Check sheet for the drawn part. Datum: minimum x, y, z corner. Units: mm. Give positions to 0.01 mm unless a question says otherwise; leave off trailing zeros. Write each loop counter-clockwise with the first axis right and the second up, starting at its lowest first coordinate (ties: lowest second). Pieces come first, ordered by that corner, then holes. Notation, with made-up numbers: (-20.75, 24.5) -> (-9.75, 24.5) arc R18 ccw to (-9.75, 56.5) -> close; hole circle Ø3 at (68.5, 31.25). An arc over 180 degrees is marked (long way). Answer as CSV lines item,"result". Start each with the question number.
1) Sectioned sample at B-B on x = 38. Record the cut outline in (y, z), and give its area (3 significant figures).
2) Sectioned sample at A-A on z = 31. Record the cut outline in (x, y).
3) Material ranges on L1, parallel to X at y = 4.4, z = 39; L2, parallel to Z at x = 42.5, y = 3.35; L3, parallel to Z at x = 30.5, y = 1.75, recorded low to high.
4) Gauge pin test, flat ends, axial feed: pin 1 Ø1.5 at (x, y) = (46.5, 1.5) entering from +Z; pin 2 Ø1 at (y, z) = (2, 7.5) entering from -X; pin 3 Ø1.5 at (x, y) = (25, 2) entering from +Z. Record the tip position at first contact, or that the pin passes through.
5) Sectioned sample at C-C on y = 2.1. Record the cut outline in (x, z), and give its area (3 significant figures).
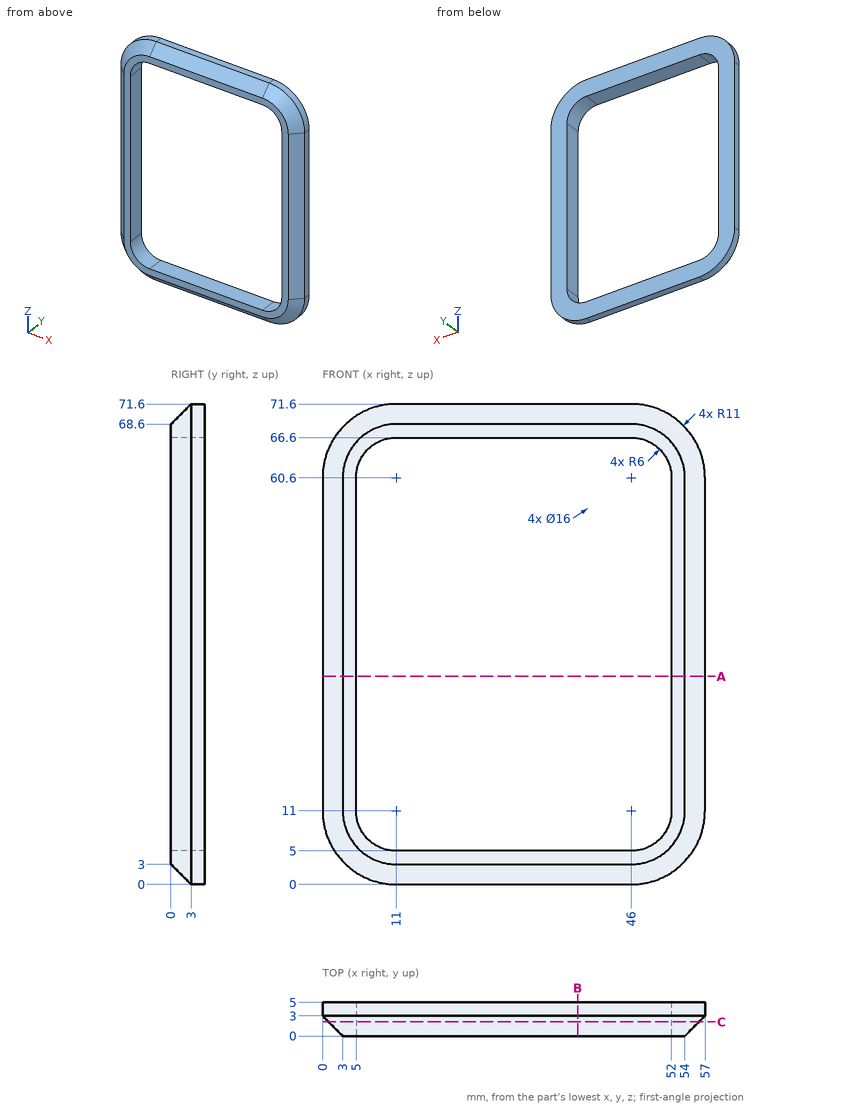
Ans:
1,outline,"(0, 3) -> (3, 0) -> (5, 0) -> (5, 5) -> (0, 5) -> close; (0, 66.6) -> (5, 66.6) -> (5, 71.6) -> (3, 71.6) -> (0, 68.6) -> close"
1,area,"41.0 mm²"
2,outline,"(0, 3) -> (3, 0) -> (5, 0) -> (5, 5) -> (0, 5) -> close; (52, 0) -> (54, 0) -> (57, 3) -> (57, 5) -> (52, 5) -> close"
3,L1,"x = 0 to 5, 52 to 57"
3,L2,"z = 0 to 5, 66.6 to 71.6"
3,L3,"z = 1.25 to 5, 66.6 to 70.35"
4,pin 1,"stops at z = 70.84"
4,pin 2,"stops at x = 1.07"
4,pin 3,"stops at z = 71.35"
5,outline,"(0.9, 11) arc R10.1 ccw to (11, 0.9) -> (46, 0.9) arc R10.1 ccw to (56.1, 11) -> (56.1, 60.6) arc R10.1 ccw to (46, 70.7) -> (11, 70.7) arc R10.1 ccw to (0.9, 60.6) -> close; hole (5, 11) arc R6 ccw to (11, 5) -> (46, 5) arc R6 ccw to (52, 11) -> (52, 60.6) arc R6 ccw to (46, 66.6) -> (11, 66.6) arc R6 ccw to (5, 60.6) -> close"
5,area,"901 mm²"
